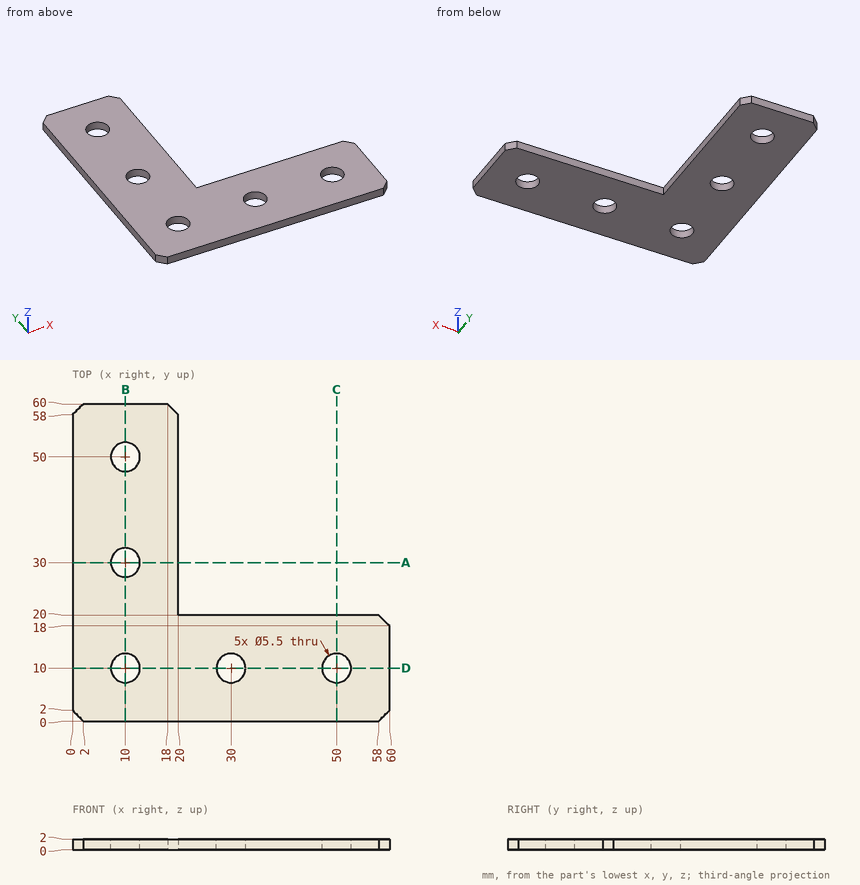
Design review of the part shown in the three views and the two pictorial views. Dimensions are in mm from the part's minimum x, y and z. Round coordinates to 2 decimals unless told otherwise and drop trailing zeros. Write each loop counter-clockwise with the first axis right and the second up, starting at its lowest first coordinate (ties: lowest second). Pieces come first, ordered by that corner, then holes.
Item 1: Consider section A-A on y = 30. Give the boundary of the cut face in (x, z).
Item 2: Consider section B-B on x = 10. Give the boundary of the cut face in (y, z), and give its area (3 significant figures).
Item 3: For pin 1 Ø0.6 at (y, z) = (36.5, 1) entering from +X, flat-tipped, find the tip position at first contact; note if it passes through.
Item 4: Wall thickness on L1, parallel to Y at x = 10, z = 0.7; L2, parallel to X at y = 50, z = 1.4: over which ranges is each line inside the solid? List them lowest first.
Check values:
1. outline: (0, 0) - (7.25, 0) - (7.25, 2) - (0, 2) - close; (12.75, 0) - (20, 0) - (20, 2) - (12.75, 2) - close
2. outline: (0, 0) - (7.25, 0) - (7.25, 2) - (0, 2) - close; (12.75, 0) - (27.25, 0) - (27.25, 2) - (12.75, 2) - close; (32.75, 0) - (47.25, 0) - (47.25, 2) - (32.75, 2) - close; (52.75, 0) - (60, 0) - (60, 2) - (52.75, 2) - close
2. area: 87.0 mm2
3. pin 1: stops at x = 20
4. L1: y = 0 to 7.25, 12.75 to 27.25, 32.75 to 47.25, 52.75 to 60
4. L2: x = 0 to 7.25, 12.75 to 20
